Could you check a few things on this model? Use its own coordinates, in mm. Face numbers are marked on the shaded views. A direction names the side the tool comes from. Round coordinates to 2 decimals unless told otherwise and drop trailing zeros. Write each loop counter-clockwise with the first axis right and the second up, starting at its lowest first coordinate (ties: lowest second). Pieces come first, ordered by that corner, then holes. Notation, with made-up numbers: M 63,-5.75 L 72,-5.75 A25 ccw 72,24.25 Z; hole C 39.25,70.5 d8. An arc over 180 degrees is marked long. One line per item, written item: value. Start each with the question number.
(1) I want a section at A-A on z = -17.5. Please give me the cut outline in (x, y), and give its area (3 significant figures).
(2) If I drill on L1, parallel to Y at x = 3.55, z = -17.75; L2, parallel to Z at x = 3.9, y = -1.25; L3, parallel to Z at x = 1.8, y = 1.25, over which ranges is the centre line in solid material (lowest first)?
(3) I want a section at C-C on y = -0.5. Please give me the cut outline in (x, z).
(4) Thinking about a two-plate mould opening in Z: for the marked faces 3, 4 and 5, which applies, released by +Z, released by -Z, zero draft, split by the parting line, or undercut?
(5) I want a section at D-D on y = 4.25. Please give me the cut outline in (x, z).
(6) Which directions (+Z, -Z, +X, -X, +Y, -Y) give clear straight access to the entire face, cutting with the end or side of a thin tool? Please do the marked faces 1 and 2.
(7) I want a section at B-B on x = 0.45. Please give me the cut outline in (y, z).
(8) I'm going to push a flat-ended pin straight in: pin 1 Ø1 at (x, y) = (0.5, 3) entering from +Z. Where does the tip first touch, or does it pass through?
```python
from build123d import *

# Parameters (mm, degrees)
BOSS_EXTRUDE1_DEPTH = 5
CUT_EXTRUDE1_DEPTH  = 23.867116988


with BuildPart() as part:
    # Sketch1 → Boss-Extrude1 (new body)
    with BuildSketch(Plane(origin=(0, 0, 0), x_dir=(0, 0, -1), z_dir=(1, 0, 0))):
        Polygon((0, 6), (0, -6), (18.812364002, -6), (18.812364002, -3), (13.95008688, -3), (13.95008688, 3), (18.812364002, 3), (18.812364002, 6), align=None)
    extrude(amount=BOSS_EXTRUDE1_DEPTH)

    # Sketch2 → Cut-Extrude1 (cut, through all)
    with BuildSketch(Plane(origin=(0, 6, 0), x_dir=(1, 0, 0), z_dir=(0, 1, 0))):
        Polygon((0, 4), (0, 0), (2.5, 0), align=None)
    extrude(amount=-CUT_EXTRUDE1_DEPTH, mode=Mode.SUBTRACT)


solid = part.part
```
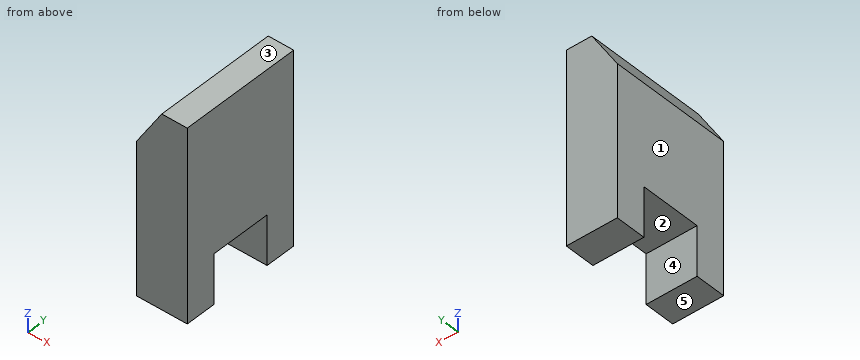
Found:
1. outline: M 0,-6 L 5,-6 L 5,-3 L 0,-3 Z; M 0,3 L 5,3 L 5,6 L 0,6 Z
1. area: 30.0 mm²
2. L1: y = -6 to -3, 3 to 6
2. L2: z = -13.95 to 0
2. L3: z = -13.95 to -1.12
3. outline: M 0,-13.95 L 5,-13.95 L 5,0 L 2.5,0 L 0,-4 Z
4. face 3: released by +Z
4. face 4: zero draft
4. face 5: released by -Z
5. outline: M 0,-18.81 L 5,-18.81 L 5,0 L 2.5,0 L 0,-4 Z
6. face 1: +Z, -Z, -X, +Y, -Y
6. face 2: -Z, +X, -X
7. outline: M -6,-18.81 L -3,-18.81 L -3,-13.95 L 3,-13.95 L 3,-18.81 L 6,-18.81 L 6,-3.28 L -6,-3.28 Z
8. pin 1: stops at z = -2.4
